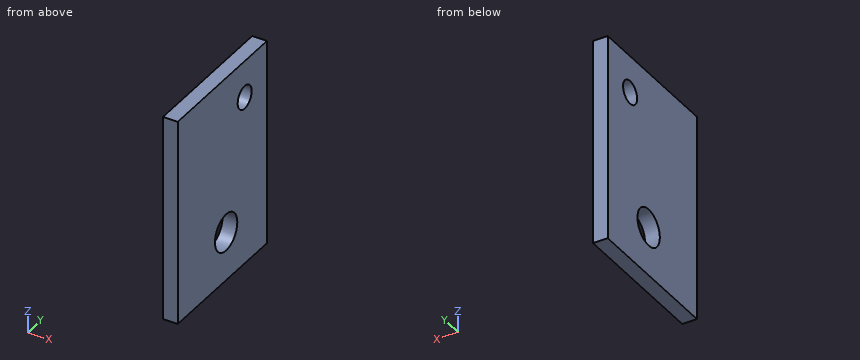
Autodesk Inventor part; units mm, degrees
ref_plane "YZ Plane" through (0, 0, 0) normal (1, 0, 0) x (0, 1, 0)
ref_plane "XZ Plane" through (0, 0, 0) normal (0, 1, 0) x (-1, 0, 0)
ref_plane "XY Plane" through (0, 0, 0) normal (0, 0, 1) x (1, 0, 0)
sketch "Sketch1" plane through (0, 0, 0) normal (1, 0, 0) x (0, 1, 0)
  circle A0 centre (-6.35, -6.35) radius 1.9939
  circle A1 centre (-11.6332, -27.1526) radius 3.175
  line L0 (0, 0) -> (-25.4, 0)
  line L1 (-25.4, 0) -> (-25.4, -35.56)
  line L2 (-25.4, -35.56) -> (0, -35.56)
  line L3 (0, -35.56) -> (0, 0)
  dimension "d2" = 3.9878
  dimension "d5" = 6.35
  dimension "d6" = 25.4
  dimension "d7" = 35.56
extrude "Extrusion1" add sketch "Sketch1" along normal blind 2.54
properties part number "mounting bracket"
Could you check a few things on this model? Use its own coordinates, in mm. Round coordinates to 2 decimals unless told otherwise and drop trailing zeros. Write each loop counter-clockwise with the first axis right and the second up, starting at its lowest first coordinate (ties: lowest second). Pieces come first, ordered by that corner, then holes. Notation, with made-up numbers: (30, 75.5) -> (78, 75.5) arc R7 ccw to (78, 85.5) -> close; hole circle Ø11 at (21.5, -2). An arc over 180 degrees is marked (long way). Use a Markdown table: item, result.
1. For pin 1 Ø3.5 at (y, z) = (-6.35, -6.35) entering from +X, with a flat end and sliding along its axis, tell me the tip position at first contact or that it passes through.
Answer key:
| item | result |
|---|---|
| pin 1 | passes through |
2. Please list where these lines run through material, in increasing order: probe 1 along Z at (x, y) = (1.65, -6.35); probe 2 along Z at (x, y) = (1.55, -11); probe 3 along Y at (x, z) = (0.4, -26).
Answer key:
| item | result |
|---|---|
| probe 1 | z = -35.56 to -8.34, -4.36 to 0 |
| probe 2 | z = -35.56 to -30.26, -24.04 to 0 |
| probe 3 | y = -25.4 to -14.59, -8.67 to 0 |
3. If we section it at A-A (y = -6.35): List the corners of the cut face in (x, z) for me, then the cut area to 3 significant figures.
Answer key:
| item | result |
|---|---|
| outline | (0, -35.56) -> (2.54, -35.56) -> (2.54, -8.34) -> (0, -8.34) -> close; (0, -4.36) -> (2.54, -4.36) -> (2.54, 0) -> (0, 0) -> close |
| area | 80.2 mm^2 |
4. If we section it at C-C (x = 1.7): List the corners of the cut face in (y, z) for me (3 decimals), then the cut area to 3 significant figures.
Answer key:
| item | result |
|---|---|
| outline | (-25.4, -35.56) -> (0, -35.56) -> (0, 0) -> (-25.4, 0) -> close; hole circle Ø6.35 at (-11.633, -27.153); hole circle Ø3.988 at (-6.35, -6.35) |
| area | 859 mm^2 |
5. If we section it at B-B (z = -6.35): List the corners of the cut face in (x, y) for me.
Answer key:
| item | result |
|---|---|
| outline | (0, -25.4) -> (2.54, -25.4) -> (2.54, -8.34) -> (0, -8.34) -> close; (0, -4.36) -> (2.54, -4.36) -> (2.54, 0) -> (0, 0) -> close |
